from build123d import *

# Parameters (mm, degrees)
SKETCH1_R           = 3.5
BOSS_EXTRUDE1_DEPTH = 16
SKETCH2_R           = 1
BOSS_EXTRUDE2_DEPTH = 0.5
SKETCH3_R           = 0.5
BOSS_EXTRUDE3_DEPTH = 4
FILLET1_R           = 0.25
SKETCH7_R           = 3.475
BOSS_EXTRUDE6_DEPTH = 0.5
BOSS_EXTRUDE7_START = 1
SKETCH8_R           = 1
BOSS_EXTRUDE7_DEPTH = 1


with BuildPart() as part:
    # Sketch1 → Boss-Extrude1 (new body)
    with BuildSketch(Plane(origin=(0, 0, 0), x_dir=(0, 0, -1), z_dir=(1, 0, 0))):
        Circle(SKETCH1_R)
    extrude(amount=-BOSS_EXTRUDE1_DEPTH)

    # Sketch2 → Boss-Extrude2 (add)
    with BuildSketch(Plane(origin=(0, 0, 0), x_dir=(0, 0, -1), z_dir=(1, 0, 0))):
        Circle(SKETCH2_R)
    extrude(amount=BOSS_EXTRUDE2_DEPTH)

    # Sketch3 → Boss-Extrude3 (add)
    with BuildSketch(Plane(origin=(0.5, 0, 0), x_dir=(0, 0, -1), z_dir=(1, 0, 0))):
        Circle(SKETCH3_R)
    extrude(amount=BOSS_EXTRUDE3_DEPTH)

    # Fillet1
    fillet1_edges = [part.edges().sort_by_distance(p)[0] for p in [
        (4.5, 0, 0.5),
    ]]
    fillet(fillet1_edges, radius=FILLET1_R)

    # Sketch7 → Boss-Extrude6 (add)
    with BuildSketch(Plane.ZY.offset(16)):
        with Locations(Location((0, 0, 0), (0, 0, 180))):
            Circle(SKETCH7_R)
    extrude(amount=BOSS_EXTRUDE6_DEPTH)

    # Sketch8 → Boss-Extrude7 (add)
    with BuildSketch(Plane.ZY.offset(16.5).offset(BOSS_EXTRUDE7_START)):
        with Locations(Location((0, 0, 0), (0, 0, 180))):
            Circle(SKETCH8_R)
    extrude(amount=-BOSS_EXTRUDE7_DEPTH)


solid = part.part
Could you check a few things on this model? Use its own coordinates, in mm. A direction names the side the tool comes from. Give positions to 0.01 mm unless a question says otherwise; leave off trailing zeros. Loops run counter-clockwise (first coordinate to the right, second up) from the corner with the lowest first, then second, coordinate; pieces in that order, holes last. Notation, with made-up numbers: M -35,27.25 L 18,27.25 A17 cw 18,32.25 Z; hole C 59.25,10 d5. An arc over 180 degrees is marked long. Answer as a JSON object with one key per item and string values.
Q1. Suppose I cut it at C-C, the plane x = -7. List the corners of the cut face in (y, z) for me, plus the area to 3 significant figures.
Values found:
{"outline": "C 0,0 d7", "area": "38.5 mm²"}
Q2. For P1, Ø2, axis at x = 1.5, y = -2, coming from the +Z side; P2, Ø2, axis at x = -12.5, z = 2, coming from the -Y side; P3, Ø2, axis at y = -1.5, z = -0.5, coming from the +X side; P4, Ø1, axis at x = -7.5, z = -2, coming from the +Y side, each with a flat end and sliding along its axis, tell me the tip position at first contact or that it passes through.
Values found:
{"P1": "passes through", "P2": "stops at y = -3.35", "P3": "stops at x = 0.5", "P4": "stops at y = 3.16"}
Q3. For faces 1 (the flat face through (-17.5, 0, 0)), 2 (the cylindrical face through (-17, 1, 0)), 3 (the cylindrical face through (2.349, -0.488, 0.108)), which set-ups out of +Z, -Z, +X, -X, +Y, -Y let a thin tool reach every point of the face, with its end or its side?
Values found:
{"face 1": "+Z, -Z, -X, +Y, -Y", "face 2": "-X", "face 3": "+X"}
Q4. If I drill on probe 1 along X at (y, z) = (1.25, 2.25); probe 2 along Z at (x, y) = (-16.25, -0.75); probe 3 along Z at (x, y) = (-7.25, 0.25), over which ranges is the centre line in solid material (lowest first)? Write a range as [from, to].
Values found:
{"probe 1": "x = [-16.5, 0]", "probe 2": "z = [-3.39, 3.39]", "probe 3": "z = [-3.49, 3.49]"}
Q5. Suppose I cut it at A-A, the plane z = 3.25. List the corners of the cut face in (x, y) for me, plus the area to 3 significant figures.
Values found:
{"outline": "M -16.5,-1.23 L -16,-1.23 L -16,-1.3 L 0,-1.3 L 0,1.3 L -16,1.3 L -16,1.23 L -16.5,1.23 Z", "area": "42.8 mm²"}
Q6. Suppose I cut it at D-D, the plane x = 1.5. List the corners of the cut face in (y, z) for me.
Values found:
{"outline": "C 0,0 d1"}
